from build123d import *

# Parameters (mm, degrees)
SKETCH1_R               = 9
SKETCH1_R_2             = 4
BOSS_EXTRUDE1_DEPTH     = 27
SKETCH2_R               = 9
SKETCH2_R_2             = 6
CUT_EXTRUDE1_DEPTH      = 0.5
SKETCH3_R               = 1.5
CUT_EXTRUDE2_DEPTH      = 10
CUT_EXTRUDE2_DEPTH_BACK = 10
SKETCH4_R               = 4
BOSS_EXTRUDE2_DEPTH     = 5


with BuildPart() as part:
    # Sketch1 → Boss-Extrude1 (new body)
    with BuildSketch(Plane(origin=(0, 0, 0), x_dir=(1, 0, 0), z_dir=(0, 1, 0))):
        Circle(SKETCH1_R)
        Circle(SKETCH1_R_2, mode=Mode.SUBTRACT)
    extrude(amount=BOSS_EXTRUDE1_DEPTH)

    # Sketch2 → Cut-Extrude1 (cut)
    with BuildSketch(Plane(origin=(0, 27, 0), x_dir=(1, 0, 0), z_dir=(0, 1, 0))):
        Circle(SKETCH2_R)
        Circle(SKETCH2_R_2, mode=Mode.SUBTRACT)
    extrude(amount=-CUT_EXTRUDE1_DEPTH, mode=Mode.SUBTRACT)

    # Sketch3 → Cut-Extrude2 (cut, two sides)
    with BuildSketch(Plane.XY) as cut_extrude2_sk:
        with Locations((0, 19.5)):
            Circle(SKETCH3_R)
    extrude(amount=CUT_EXTRUDE2_DEPTH, mode=Mode.SUBTRACT)
    extrude(cut_extrude2_sk.sketch, amount=-CUT_EXTRUDE2_DEPTH_BACK, mode=Mode.SUBTRACT)

    # Sketch4 → Boss-Extrude2 (add)
    with BuildSketch(Plane(origin=(0, 14.5, 0), x_dir=(1, 0, 0), z_dir=(0, 1, 0))):
        Polygon((13.279056191, 0), (6.639528096, 11.5), (-6.639528096, 11.5), (-13.279056191, 0), (-6.639528096, -11.5), (6.639528096, -11.5), align=None)
        Circle(SKETCH4_R, mode=Mode.SUBTRACT)
    extrude(amount=-BOSS_EXTRUDE2_DEPTH)


solid = part.part
Verification items for the finished model (mm, model axes). A direction names the side the tool comes from. Give positions to 0.01 mm unless a question says otherwise; leave off trailing zeros. Write each loop counter-clockwise with the first axis right and the second up, starting at its lowest first coordinate (ties: lowest second). Pieces come first, ordered by that corner, then holes.
(1) Cross-section at B-B (y = 13.75). Enter the section's corners in (x, z).
(2) Material ranges on line 1 (Y direction, x = 0, z = -4.75); line 2 (Y direction, x = 0, z = 6.6); line 3 (X direction, y = 21, z = 0), recorded low to high.
(3) Access from +Z, -Z, +X, -X, +Y, -Y to the whole of each face (thin tool, end or side, straight path). Record for faces 5 (the face through (2, 26.5, 6)), 6 (the face through (-1.172, 4.684, -8.923)), 7 (the face through (-9.913, 12.035, -5.83)).
(4) Cross-section at D-D (y = 19.5). Enter the section's corners in (x, z), plus the area to 3 significant figures.
(5) Mould release check, pull along Z, two halves, no side actions. Record for faces 1 (the face through (-10.006, 12.035, 5.67)), 2 (the face through (3.695, 13.311, 1.532)), 3 (the face through (4, 0, 2)), 4 (the face through (0, 12, -11.5)): +Z half, -Z half, draft (parallel to the pull), parting line (faces both ways), or undercut.
(6) Cross-section at A-A (x = 0). Enter the section's corners in (y, z).
(7) Gauge pin test, flat ends, axial feed: pin 1 (4 mm diameter, centred on y = 16, z = -6, fed in from -X); pin 2 (5 mm diameter, centred on x = 0, y = 19.5, fed in from -Z). Record the tip position at first contact, or that the pin passes through.
(8) Cross-section at C-C (z = 1.75). Enter the section's corners in (x, y), plus the area to 3 significant figures.
Worked out:
1. outline: (-13.28, 0) - (-6.64, -11.5) - (6.64, -11.5) - (13.28, 0) - (6.64, 11.5) - (-6.64, 11.5) - close; hole circle Ø8 at (0, 0)
2. line 1: y = 0 to 18, 21 to 27
2. line 2: y = 0 to 18, 21 to 26.5
2. line 3: x = -9 to -4, 4 to 9
3. face 5: +Y
3. face 6: -Y
3. face 7: -Z, -X, +Y, -Y
4. outline: (-1.5, -8.87) - (-1.5, -3.71) arc R4 cw to (-1.5, 3.71) - (-1.5, 8.87) arc R9 ccw to start; (1.5, -8.87) arc R9 ccw to (1.5, 8.87) - (1.5, 3.71) arc R4 cw to (1.5, -3.71) - close
4. area: 174 mm2
5. face 1: +Z half
5. face 2: undercut
5. face 3: draft
5. face 4: -Z half
6. outline: (0, -9) - (9.5, -9) - (9.5, -11.5) - (14.5, -11.5) - (14.5, -9) - (18, -9) - (18, -4) - (0, -4) - close; (0, 4) - (18, 4) - (18, 9) - (14.5, 9) - (14.5, 11.5) - (9.5, 11.5) - (9.5, 9) - (0, 9) - close; (21, -9) - (26.5, -9) - (26.5, -6) - (27, -6) - (27, -4) - (21, -4) - close; (21, 4) - (27, 4) - (27, 6) - (26.5, 6) - (26.5, 9) - (21, 9) - close
7. pin 1: stops at x = -10.58
7. pin 2: stops at z = -9
8. outline: (-12.27, 9.5) - (-8.83, 9.5) - (-8.83, 0) - (-3.6, 0) - (-3.6, 27) - (-5.74, 27) - (-5.74, 26.5) - (-8.83, 26.5) - (-8.83, 14.5) - (-12.27, 14.5) - close; (3.6, 0) - (8.83, 0) - (8.83, 9.5) - (12.27, 9.5) - (12.27, 14.5) - (8.83, 14.5) - (8.83, 26.5) - (5.74, 26.5) - (5.74, 27) - (3.6, 27) - close
8. area: 314 mm2
